```python
from build123d import *

# Parameters (mm, degrees)
SKETCH1_W            = 688.1
SKETCH1_H            = 688.1
SKETCH1_W_2          = 650
SKETCH1_H_2          = 650
BOSS_EXTRUDE1_DEPTH  = 661.9
SKETCH3_W            = 25.4
SKETCH3_H            = 650
CUT_EXTRUDE1_DEPTH   = 9.525
SKETCH4_W            = 25.4
SKETCH4_H            = 669.5
SKETCH4_H_2          = 669.05
CUT_EXTRUDE3_DEPTH   = 9.525
SKETCH6_W            = 25.4
SKETCH6_H            = 669.5
CUT_EXTRUDE4_DEPTH   = 9.525
CUT_EXTRUDE5_DEPTH   = 700
MIRROR6_COPY_1_DEPTH = 700


with BuildPart() as part:
    # Sketch1 → Boss-Extrude1 (new body)
    with BuildSketch(Plane(origin=(0, 0, 0), x_dir=(0, 0, -1), z_dir=(1, 0, 0))):
        with Locations((344.05, 344.05)):
            Rectangle(SKETCH1_W, SKETCH1_H)
        with Locations((344.05, 344.05)):
            Rectangle(SKETCH1_W_2, SKETCH1_H_2, mode=Mode.SUBTRACT)
    extrude(amount=BOSS_EXTRUDE1_DEPTH)

    # Sketch3 → Cut-Extrude1 (cut)
    with BuildSketch(Plane.XY.offset(-669.05)):
        with Locations((168.65, 344.05)):
            Rectangle(SKETCH3_W, SKETCH3_H)
        with Locations((350, 344.05)):
            Rectangle(SKETCH3_W, SKETCH3_H)
        with Locations((531.35, 344.05)):
            Rectangle(SKETCH3_W, SKETCH3_H)
    cut_extrude1 = extrude(amount=-CUT_EXTRUDE1_DEPTH, mode=Mode.SUBTRACT)

    # Mirror2: Cut-Extrude1 across plane
    add(cut_extrude1.mirror(Plane(origin=(0, 0, -344.05), x_dir=(1, 0, 0), z_dir=(0, 0, -1))), mode=Mode.SUBTRACT)

    # Sketch4 → Cut-Extrude3 (cut)
    with BuildSketch(Plane(origin=(0, 19.05, 0), x_dir=(1, 0, 0), z_dir=(0, 1, 0))):
        with Locations((168.65, 343.825)):
            Rectangle(SKETCH4_W, SKETCH4_H)
        with Locations((350, 343.825)):
            Rectangle(SKETCH4_W, SKETCH4_H)
        with Locations((531.35, 344.05)):
            Rectangle(SKETCH4_W, SKETCH4_H_2)
    cut_extrude3 = extrude(amount=-CUT_EXTRUDE3_DEPTH, mode=Mode.SUBTRACT)

    # Mirror4: Cut-Extrude3 across plane
    add(cut_extrude3.mirror(Plane.ZX.offset(344.05)), mode=Mode.SUBTRACT)

    # Sketch6 → Cut-Extrude4 (cut)
    with BuildSketch(Plane(origin=(0, 688.1, 0), x_dir=(1, 0, 0), z_dir=(0, 1, 0))):
        with Locations((168.65, 344.275)):
            Rectangle(SKETCH6_W, SKETCH6_H)
        with Locations((350, 343.825)):
            Rectangle(SKETCH6_W, SKETCH6_H)
        with Locations((531.35, 343.825)):
            Rectangle(SKETCH6_W, SKETCH6_H)
    extrude(amount=-CUT_EXTRUDE4_DEPTH, mode=Mode.SUBTRACT)

    # Sketch7 → Cut-Extrude5 (cut)
    with BuildSketch(Plane.ZY):
        Polygon((-19.05, 39.05), (-9.525, 39.05), (-9.525, 9.525), (-39.05, 9.525), (-39.05, 19.05), (-19.05, 19.05), align=None)
    cut_extrude5 = extrude(amount=-CUT_EXTRUDE5_DEPTH, mode=Mode.SUBTRACT)

    # Mirror5: Cut-Extrude5 across plane
    add(cut_extrude5.mirror(Plane(origin=(0, 0, -344.05), x_dir=(1, 0, 0), z_dir=(0, 0, -1))), mode=Mode.SUBTRACT)

    # Mirror6: Cut-Extrude5 across plane
    add(cut_extrude5.mirror(Plane.ZX.offset(344.05)), mode=Mode.SUBTRACT)

    # Mirror6 copy 1 sketch → Mirror6 copy 1 (cut)
    with BuildSketch(Plane(origin=(0, 688.1, -688.1), x_dir=(0, 0, -1), z_dir=(-1, 0, 0))):
        Polygon((-19.05, 39.05), (-9.525, 39.05), (-9.525, 9.525), (-39.05, 9.525), (-39.05, 19.05), (-19.05, 19.05), align=None)
    extrude(amount=-MIRROR6_COPY_1_DEPTH, mode=Mode.SUBTRACT)


solid = part.part
```
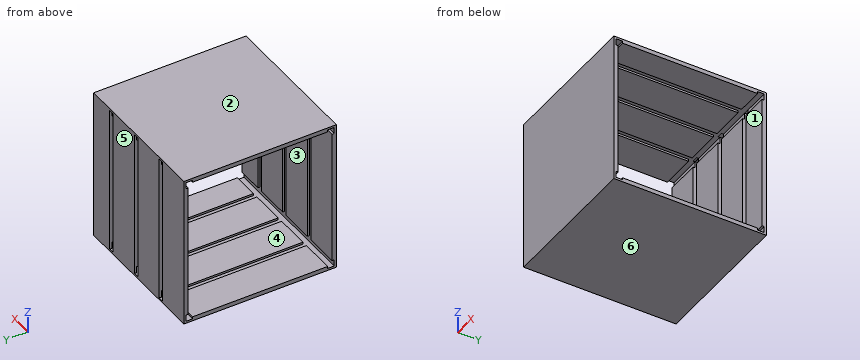
Read the model definition and answer for the solid it produces. Units are mm, in the model's axes. Face numbers are marked on the shaded views. A direction names the side the tool comes from. Give positions to 0.01 mm unless a question says otherwise; leave off trailing zeros. Write each loop counter-clockwise with the first axis right and the second up, starting at its lowest first coordinate (ties: lowest second). Pieces come first, ordered by that corner, then holes. Notation, with made-up numbers: M -31,70 L 1,70 A10 ccw 1,76 Z; hole C -16.5,-23 d2. An arc over 180 degrees is marked long. Put each result on its own line as item: value. Start each with the question number.
1. The part is cut by section A-A, the plane x = 401.5. Give the vertices of the cut face in (y, z) (3 decimals), and give its area (3 significant figures).
2. Consider line 1 along Z through (x, y) = (519.5, 483) (3 decimals); line 2 along Y through (x, z) = (53, -160); line 3 along Z through (x, y) = (198, 376.5). Determine where each line is inside the solid, lowest interval first.
3. For a pull along Y with two mould halves and no side action, classify the marked faces 3, 4, 5 and 6 as released by +Y, released by -Y, zero draft, split by the parting line, or undercut.
4. This flat-tipped pin is pushed along its axis until it touches: pin 1 Ø4 at (x, z) = (361, -583) entering from +Y. Where does it stop, or does it pass through?
5. Which of the six approach directions +Z, -Z, +X, -X, +Y, -Y give full straight-line access (tool end or side, diameter ignored) to the marked faces 1 and 2?
6. The part is cut by section B-B, the plane z = -76. Give the number of separate pieces and of enclosed holes in the cut face, and give its area (3 significant figures).
Final values:
1. outline: M 0,-688.1 L 688.1,-688.1 L 688.1,0 L 0,0 Z; hole M 9.525,-678.575 L 39.05,-678.575 L 39.05,-669.05 L 649.05,-669.05 L 649.05,-678.575 L 678.575,-678.575 L 678.575,-649.05 L 669.05,-649.05 L 669.05,-39.05 L 678.575,-39.05 L 678.575,-9.525 L 649.05,-9.525 L 649.05,-19.05 L 39.05,-19.05 L 39.05,-9.525 L 9.525,-9.525 L 9.525,-39.05 L 19.05,-39.05 L 19.05,-649.05 L 9.525,-649.05 Z
1. area: 49,100 mm²
2. line 1: z = -688.1 to -678.575, -9.525 to 0
2. line 2: y = 0 to 19.05, 669.05 to 688.1
2. line 3: z = -688.1 to -669.05, -19.05 to 0
3. face 3: undercut
3. face 4: undercut
3. face 5: released by +Y
3. face 6: zero draft
4. pin 1: stops at y = 688.1
5. face 1: +X, -X
5. face 2: +Z, +X, -X, +Y, -Y
6. separate pieces: 5
6. enclosed holes: 0
6. area: 23,000 mm²
